Work out the finished part from the listing and answer in its coordinate system (mm). Face numbers are marked on the shaded views. Round coordinates to 2 decimals unless told otherwise and drop trailing zeros. Order: outer loops, then holes, each group sorted by start corner. A loop starts at its lowest first (then second) coordinate and runs counter-clockwise, first axis right, second up.
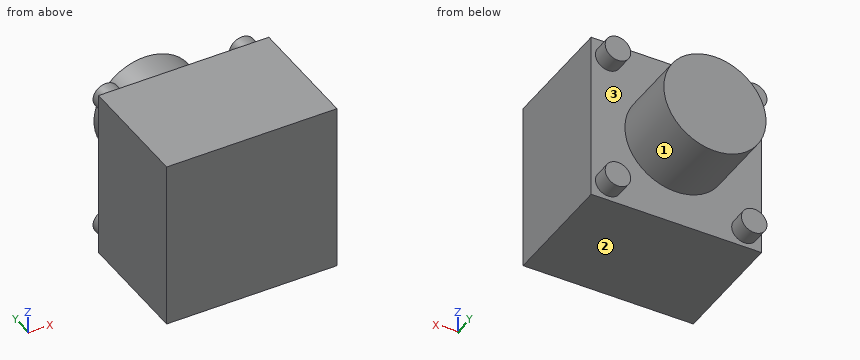
from build123d import *

# Parameters (mm, degrees)
SKETCH1_W           = 10
SKETCH1_H           = 10
BOSS_EXTRUDE1_DEPTH = 7
SKETCH3_R           = 0.75
BOSS_EXTRUDE2_DEPTH = 1
SKETCH4_R           = 3
BOSS_EXTRUDE4_DEPTH = 4


with BuildPart() as part:
    # Sketch1 → Boss-Extrude1 (new body)
    with BuildSketch(Plane(origin=(0, 0, 0), x_dir=(1, 0, 0), z_dir=(0, 1, 0))):
        with Locations((-3.108910891, -0.430693069)):
            Rectangle(SKETCH1_W, SKETCH1_H)
    extrude(amount=BOSS_EXTRUDE1_DEPTH)

    # Sketch3 → Boss-Extrude2 (add)
    with BuildSketch(Plane(origin=(0, 7, 0), x_dir=(1, 0, 0), z_dir=(0, 1, 0))):
        with Locations((-7.108910891, 3.569306931)):
            Circle(SKETCH3_R)
        with Locations((-7.108910891, -4.430693069)):
            Circle(SKETCH3_R)
        with Locations((0.891089109, -4.430693069)):
            Circle(SKETCH3_R)
        with Locations((0.891089109, 3.569306931)):
            Circle(SKETCH3_R)
    extrude(amount=BOSS_EXTRUDE2_DEPTH)

    # Sketch4 → Boss-Extrude4 (add)
    with BuildSketch(Plane(origin=(0, 7, 0), x_dir=(1, 0, 0), z_dir=(0, 1, 0))):
        with Locations((-3.088623083, -0.430693069)):
            Circle(SKETCH4_R)
    extrude(amount=BOSS_EXTRUDE4_DEPTH)


solid = part.part
Item 1: Find the intervals of material crossed by line 1 along Y through (x, z) = (-6.25, 2); line 2 along Y through (x, z) = (1, 4.5); line 3 along X through (y, z) = (10.5, -0.75), in increasing order.
Item 2: Find section D-D (z = -3.25). Write down the section's boundary in (x, y).
Item 3: For a pull along Z with two mould halves and no side action, classify the marked faces 1, 2 and 3 as released by +Z, released by -Z, zero draft, split by the parting line, or undercut.
Item 4: Find section B-B (x = -4.75). Write down the section's boundary in (y, z).
Item 5: Given pin 1 (3 mm diameter, centred on y = 7.5, z = 4, fed in from -X); pin 2 (0.8 mm diameter, centred on x = 0.5, z = 4, fed in from +Y), each flat-ended and moving along its own axis, determine where each tip first touches the part or whether it passes through.
Item 6: Find section C-C (z = -0.75). Write down the section's boundary in (x, y).
Item 7: Find section A-A (y = 7.25). Write down the section's boundary in (x, z).
Model answer:
1. line 1: y = 0 to 7
1. line 2: y = 0 to 8
1. line 3: x = -5.85 to -0.33
2. outline: (-8.11, 0) - (1.89, 0) - (1.89, 7) - (1.57, 7) - (1.57, 8) - (0.21, 8) - (0.21, 7) - (-6.43, 7) - (-6.43, 8) - (-7.79, 8) - (-7.79, 7) - (-8.11, 7) - close
3. face 1: split by the parting line
3. face 2: released by -Z
3. face 3: undercut
4. outline: (0, -4.57) - (7, -4.57) - (7, -2.07) - (11, -2.07) - (11, 2.93) - (7, 2.93) - (7, 5.43) - (0, 5.43) - close
5. pin 1: stops at x = -8.11
5. pin 2: stops at y = 8
6. outline: (-8.11, 0) - (1.89, 0) - (1.89, 7) - (-0.33, 7) - (-0.33, 11) - (-5.85, 11) - (-5.85, 7) - (-8.11, 7) - close
7. outline: circle Ø1.5 at (-7.11, -3.57); circle Ø1.5 at (-7.11, 4.43); circle Ø6 at (-3.09, 0.43); circle Ø1.5 at (0.89, -3.57); circle Ø1.5 at (0.89, 4.43)
